```python
from build123d import *

# Parameters (mm, degrees)
F0_R     = 43.8070462956
F1_DEPTH = 90.678
F2_DEPTH = 94.742
F7_DEPTH = 25.4


# Not quite as in the source:
# - the program builds the solid bodies; features that only make, move or delete a surface that nothing else refers to are left out


with BuildPart() as f1:
    # F0 (on Front) → F1 (new body)
    with BuildSketch(Plane.XZ):
        Circle(F0_R)
    extrude(amount=F1_DEPTH)

    # F2 (add): a face of the model
    f2_faces = [f1.faces().sort_by_distance(p)[0] for p in [
        (0, -90.678, 0),
    ]]
    extrude(f2_faces, amount=F2_DEPTH)

    # F4 (on Right) → F7 (join)
    with BuildSketch(Plane.YZ):
        Polygon((0, -44.503852725), (-76.628126204, -43.6692126095), (0, -76.0243907571), align=None)
    extrude(amount=F7_DEPTH)


solid = f1.part
```
Input: part model. Units: mm. Frame: model coordinates. A direction names the side the tool comes from. Coordinates: 2 decimals unless noted, no trailing zeros. Write each loop counter-clockwise with the first axis right and the second up, starting at its lowest first coordinate (ties: lowest second). Pieces come first, ordered by that corner, then holes. Notation, with made-up numbers: (-14, -27) - (6, -27) arc R22 ccw to (6, -14) - close; hole circle Ø2 at (9, -36). An arc over 180 degrees is marked (long way). Put each result on its own line as item: value. Start each with the question number.
1) Reachability of faces 3 (the face through (-1, 0, 1)), 4 (the face through (0, -22, -53)) from +Z, -Z, +X, -X, +Y, -Y: full face, straight path, thin tool, end or side. Return the list, or none.
2) Contact query for flat-ended pins moving along their axis: pin 1 (8 mm diameter, centred on y = -137.5, z = -28, fed in from +X); pin 2 (10 mm diameter, centred on y = -50, z = -16, fed in from -X); pin 3 (4 mm diameter, centred on y = -86, z = 23.5, fed in from +X). Output: stop coordinate, or through.
3) Cut plane B-B (y = -69). Return the cut outline in (x, z).
4) Cut plane C-C (x = -27). Return the cut outline in (y, z).
5) Cut plane D-D (z = 29). Return the cut outline in (x, y).
6) Ray query, L1, parallel to Z at x = 25, y = -29.5; L2, parallel to Z at x = -2, y = -140; L3, parallel to Z at x = -21.5, y = -145. Return the intervals inside material, ascending.
7) Cut plane A-A (y = -35). Return the cut outline in (x, z), plus the area to 3 significant figures.
8) Mould query, pull axis Z, two halves, no side actions, for faces 1 (the face through (25.4, -22, -52)), 2 (the face through (12.5, -38.9, -59.6)). Classes: pulls with the +Z half, pulls with the -Z half, needs draft (parallel to the pull), parting line crosses it, or undercut.
Resolved:
1. face 3: +Z, -Z, +X, -X, +Y
1. face 4: -Z, -X, +Y, -Y
2. pin 1: stops at x = 36.65
2. pin 2: stops at x = -42.4
2. pin 3: stops at x = 38.17
3. outline: (0, -46.89) - (25.4, -46.89) - (25.4, -43.75) - (2.19, -43.75) arc R43.81 ccw (long way) to (0, -43.81) - close
4. outline: (-185.42, -34.5) - (0, -34.5) - (0, 34.5) - (-185.42, 34.5) - close
5. outline: (-32.83, -185.42) - (32.83, -185.42) - (32.83, 0) - (-32.83, 0) - close
6. L1: z = -63.57 to -44.18, -35.97 to 35.97
6. L2: z = -43.76 to 43.76
6. L3: z = -38.17 to 38.17
7. outline: circle Ø87.61 at (0, 0); (0, -61.25) - (25.4, -61.25) - (25.4, -44.12) - (0, -44.12) - close
7. area: 6,460 mm2
8. face 1: needs draft
8. face 2: pulls with the -Z half
